Build history of the part. All positions in model axes, mm. A direction names the side the tool comes from. Round coordinates to 2 decimals unless told otherwise and drop trailing zeros. Order: outer loops, then holes, each group sorted by start corner. A loop starts at its lowest first (then second) coordinate and runs counter-clockwise, first axis right, second up. Notation, with made-up numbers: M 87,31 L 108,31 A31 cw 108,68 Z; hole C 57.25,21 d9. An arc over 180 degrees is marked long. One line per question, with ' | ' between items. Start each with the question number.
from build123d import *

# Parameters (mm, degrees)
BOSS_EXTRUDE1_DEPTH  = 25
SKETCH2_R            = 11.2
CUT_EXTRUDE1_DEPTH   = 77.347887987
SKETCH11_W           = 90
SKETCH11_H           = 30
CUT_EXTRUDE4_DEPTH   = 15
BOSS_EXTRUDE2_DEPTH  = 10
BOSS_EXTRUDE3_DEPTH  = 10
SKETCH14_R           = 11.4
SKETCH14_R_2         = 10.4
BOSS_EXTRUDE4_DEPTH  = 3
CHAMFER1_SIZE        = 1
M5_CLEARANCE_HOLE1_D = 5.5


with BuildPart() as part:
    # Sketch1 → Boss-Extrude1 (new body)
    with BuildSketch(Plane.XY):
        with BuildLine():
            Line((50, 0), (50, 10))
            Line((50, 10), (35, 10))
            Line((35, 10), (35, 52))
            Line((35, 52), (-35, 52))
            Line((-35, 52), (-35, 10))
            Line((-35, 10), (-50, 10))
            Line((-50, 10), (-50, 0))
            Line((-50, 0), (-7.7, 0))
            Line((-7.7, 0), (-7.7, 14.560093328))
            ThreePointArc((-7.7, 14.560093328), (-6.985367881, 16.285367881), (-5.260093328, 17))
            Line((-5.260093328, 17), (5.7, 17))
            ThreePointArc((5.7, 17), (7.114213562, 16.414213562), (7.7, 15))
            Line((7.7, 15), (7.7, 0))
            Line((7.7, 0), (50, 0))
        make_face()
    extrude(amount=BOSS_EXTRUDE1_DEPTH)

    # Sketch2 → Cut-Extrude1 (cut, through all)
    with BuildSketch(Plane(origin=(0, 0, 0), x_dir=(-1, 0, 0), z_dir=(0, 0, -1))):
        with Locations((0, 37)):
            Circle(SKETCH2_R)
    extrude(amount=-CUT_EXTRUDE1_DEPTH, mode=Mode.SUBTRACT)

    # Sketch11 → Cut-Extrude4 (cut)
    with BuildSketch(Plane.XY.offset(25)):
        with Locations((0, 40)):
            Rectangle(SKETCH11_W, SKETCH11_H)
    extrude(amount=-CUT_EXTRUDE4_DEPTH, mode=Mode.SUBTRACT)

    # Sketch12 → Boss-Extrude2 (add)
    with BuildSketch(Plane.ZY.offset(35)):
        Polygon((10, 52), (10, 25), (25, 25), align=None)
    extrude(amount=-BOSS_EXTRUDE2_DEPTH)

    # Sketch13 → Boss-Extrude3 (add)
    with BuildSketch(Plane(origin=(35, 0, 0), x_dir=(0, 0, -1), z_dir=(1, 0, 0))):
        Polygon((-10, 52), (-10, 25), (-25, 25), align=None)
    extrude(amount=-BOSS_EXTRUDE3_DEPTH)

    # Sketch14 → Boss-Extrude4 (add)
    with BuildSketch(Plane.XY.offset(10)):
        with Locations((0, 37)):
            Circle(SKETCH14_R)
        with Locations((0, 37)):
            Circle(SKETCH14_R_2, mode=Mode.SUBTRACT)
    extrude(amount=-BOSS_EXTRUDE4_DEPTH)

    # Chamfer1
    # the kernel refuses this chamfer: 1 mm, written as the material it takes off along each edge
    with BuildSketch(Plane(origin=(0, 37, 7), x_dir=(1, 0, 0), z_dir=(0, -1, 0))) as chamfer1_piece_1_section:
        Polygon((10.4 + CHAMFER1_SIZE, 0), (10.4, CHAMFER1_SIZE), (10.4, 0), align=None)
    chamfer1_piece_1 = revolve(axis=Axis((0, 37, 7), (0, 0, 1)), mode=Mode.PRIVATE)
    chamfer1_piece_1 = chamfer1_piece_1 & Plane(origin=(0, 37, 7.590998704), x_dir=(-1, 0, 0), z_dir=(0, 0, -1)) * Cylinder(11.2, 46, mode=Mode.PRIVATE)
    add(chamfer1_piece_1, mode=Mode.SUBTRACT)

    # M5 Clearance Hole1 (through all)
    with Locations(Plane(origin=(0, 10, 0), x_dir=(1, 0, 0), z_dir=(0, 1, 0))):
        with Locations((42.5, -18.5), (42.5, -6.5), (-42.5, -18.5), (-42.5, -6.5)):
            Hole(M5_CLEARANCE_HOLE1_D / 2)


solid = part.part
Item 1: Cut at D-D on z = 11. Write the cut outline in (x, y).
Item 2: Flat gauge pins, fed straight in: pin 1 (12 mm diameter, centred on x = -2.5, z = 21, fed in from +Y); pin 2 (12.5 mm diameter, centred on y = 37.5, z = 10.5, fed in from +X); pin 3 (13.5 mm diameter, centred on x = 0, y = 37, fed in from -Z); pin 4 (2 mm diameter, centred on y = 39, z = 17.5, fed in from -X). Where does each tip first touch, or does it go through?
Item 3: Cut at C-C on y = 11. Write the cut outline in (x, z), then the cut area to 4 significant figures.
Item 4: Tool access for faces 1 (the face through (0, 48, 10)), 2 (the face through (30.07, 38.311, 17.605)), 3 (the face through (7.7, 8, 12)): list every direction of +Z, -Z, +X, -X, +Y, -Y with a clear straight run to the whole face (end or side of a thin tool).
Item 5: Wall check: line 1 along X through (y, z) = (5.5, 18.5); line 2 along Y through (x, z) = (0, 9); line 3 along X through (y, z) = (31, 16.5). Give the ranges that are in metal, low to high. Write a range as [from, to].
Item 6: Two-plate mould, pull along Y, no slides. Class faces 4 (the face through (-42, 10, 12)), 5 (the face through (45.247, 4.93, 18.379)), 6 (the face through (-2.255, 26.847, 9.014)): +Y half, -Y half, draft (parallel to the pull), parting line (faces both ways), or undercut.
Item 7: Cut at A-A on z = 18.5. Write the cut outline in (x, y), then the cut area to 3 significant figures.
Item 8: Cut at B-B on x = -42.5. Write the cut outline in (y, z), then the cut area to 3 significant figures.
Results found:
1) outline: M -50,0 L -7.7,0 L -7.7,14.56 A2.44 cw -5.26,17 L 5.7,17 A2 cw 7.7,15 L 7.7,0 L 50,0 L 50,10 L 35,10 L 35,50.2 L 25,50.2 L 25,25 L -25,25 L -25,50.2 L -35,50.2 L -35,10 L -50,10 Z
2) pin 1: stops at y = 25 | pin 2: stops at x = 35 | pin 3: passes through | pin 4: stops at x = -35
3) outline: M -35,0 L -7.7,0 L -7.7,25 L -35,25 Z; M 7.7,0 L 35,0 L 35,25 L 7.7,25 Z | area: 1,365 mm^2
4) face 1: +Z, +Y | face 2: +Z, +X, -X, +Y | face 3: +Z, -Z, -Y
5) line 1: x = [-50, -45.25], [-39.75, -7.7], [7.7, 39.75], [45.25, 50] | line 2: y = [17, 26.6], [47.4, 52] | line 3: x = [-35, -25], [25, 35]
6) face 4: +Y half | face 5: draft | face 6: undercut
7) outline: M -50,0 L -45.25,0 L -45.25,10 L -50,10 Z; M -39.75,0 L -7.7,0 L -7.7,14.56 A2.44 cw -5.26,17 L 5.7,17 A2 cw 7.7,15 L 7.7,0 L 39.75,0 L 39.75,10 L 35,10 L 35,36.7 L 25,36.7 L 25,25 L -25,25 L -25,36.7 L -35,36.7 L -35,10 L -39.75,10 Z; M 45.25,0 L 50,0 L 50,10 L 45.25,10 Z | area: 1,910 mm^2
8) outline: M 0,0 L 10,0 L 10,3.75 L 0,3.75 Z; M 0,9.25 L 10,9.25 L 10,15.75 L 0,15.75 Z; M 0,21.25 L 10,21.25 L 10,25 L 0,25 Z | area: 140 mm^2
